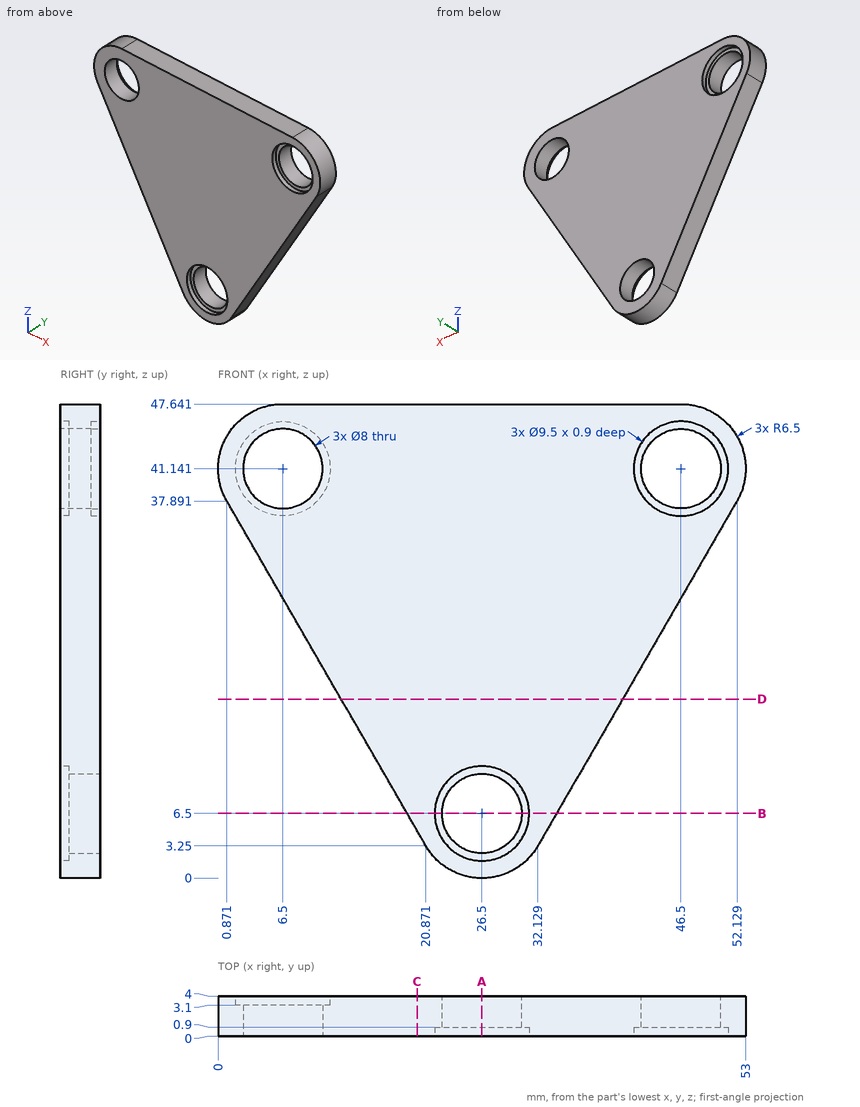
Here's the drawing with two shaded views (mm, measured from the low corner). I have some questions. Coordinates: 2 decimals unless noted, no trailing zeros. Loops run counter-clockwise (first coordinate to the right, second up) from the corner with the lowest first, then second, coordinate; pieces in that order, holes last. Notation, with made-up numbers: M 25.5,-4 L 75.5,-4 A18 cw 75.5,25 Z; hole C -7,-4 d4. An arc over 180 degrees is marked long. Put each result on its own line as item: value. Start each with the question number.
(1) Imagine slicing it at D-D on z = 18. List the corners of the cut face in (x, y) for me (3 decimals), and give its area (3 significant figures).
(2) I need wall thicknesses on probe 1 along Y at (x, z) = (46.5, 37); probe 2 along X at (y, z) = (3, 6.5) (1 decimal); probe 3 along Z at (x, y) = (19, 3.3). Which ranges of each line are inside material? Lowest first, please.
(3) Imagine slicing it at C-C on x = 20. List the corners of the cut face in (y, z) for me.
(4) Imagine slicing it at B-B on z = 6.5. List the corners of the cut face in (x, y) for me, and give its area (3 significant figures).
(5) Will these pins go through, and if not, where does the flat tip stop? pin 1 Ø5 at (x, z) = (25.5, 6.5) entering from -Y; pin 2 Ø8.5 at (x, z) = (6.5, 41.14) entering from +Y; pin 3 Ø2 at (y, z) = (1, 32) entering from +X (1 decimal); pin 4 Ø1 at (x, y) = (35.5, 3.5) entering from -Z.
(6) Imagine slicing it at A-A on x = 26.5. List the corners of the cut face in (y, z) for me, and give its area (3 significant figures).
Worked answers:
1. outline: M 12.355,0 L 40.645,0 L 40.645,4 L 12.355,4 Z
1. area: 113 mm2
2. probe 1: y = 0.9 to 4
2. probe 2: x = 19 to 22.5, 30.5 to 34
2. probe 3: z = 6.49 to 47.64
3. outline: M 0,4.76 L 4,4.76 L 4,47.64 L 0,47.64 Z
4. outline: M 18.99,0 L 21.75,0 L 21.75,0.9 L 22.5,0.9 L 22.5,4 L 18.99,4 Z; M 30.5,0.9 L 31.25,0.9 L 31.25,0 L 34.01,0 L 34.01,4 L 30.5,4 Z
4. area: 26.7 mm2
5. pin 1: passes through
5. pin 2: stops at y = 3.1
5. pin 3: stops at x = 49.3
5. pin 4: stops at z = 8.22
6. outline: M 0,0 L 4,0 L 4,2.5 L 0.9,2.5 L 0.9,1.75 L 0,1.75 Z; M 0,11.25 L 0.9,11.25 L 0.9,10.5 L 4,10.5 L 4,47.64 L 0,47.64 Z
6. area: 157 mm2
